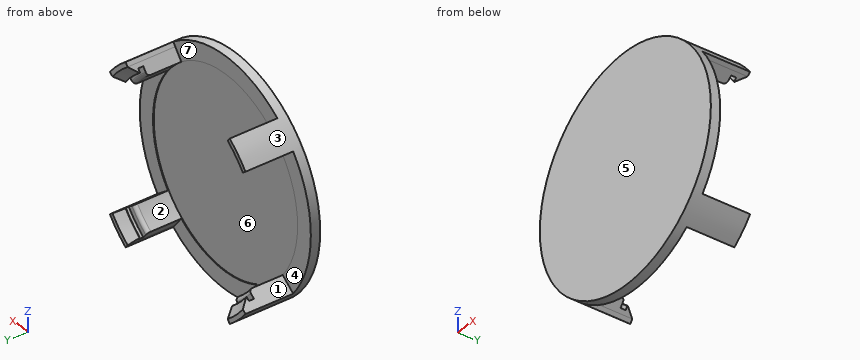
from build123d import *

# Parameters (mm, degrees)
CUT_EXTRUDE3_DEPTH = 17.4625
FILLET1_R          = 0.127
FILLET2_R          = 1.27


with BuildPart() as part:
    # Sketch1 → Revolve1 (revolve)
    with BuildSketch(Plane.XY):
        Polygon((0, 0), (-41.148, 0), (-41.148, 20.8915), (-39.5605, 20.8915), (-36.3855, 17.7165), (-37.973, 17.7165), (-37.973, 15.875), (-34.798, 15.875), (-34.798, 3.175), (0, 3.175), align=None)
    revolve(axis=Axis((0, 3.175, 0), (0, -1, 0)))

    # Sketch2 → Cut-Extrude3 (cut)
    with BuildSketch(Plane(origin=(0, 20.8915, 0), x_dir=(1, 0, 0), z_dir=(0, 1, 0))):
        with BuildLine():
            Line((-24.082906512, 31.385454819), (0, 0))
            Line((0, 0), (24.082906512, 31.385454819))
            ThreePointArc((24.082906512, 31.385454819), (0, 39.5605), (-24.082906512, 31.385454819))
        make_face()
        with BuildLine():
            Line((-25.049315281, 32.644903246), (-24.082906512, 31.385454819))
            ThreePointArc((-24.082906512, 31.385454819), (0, 39.5605), (24.082906512, 31.385454819))
            Line((24.082906512, 31.385454819), (25.049315281, 32.644903246))
            ThreePointArc((25.049315281, 32.644903246), (0, 41.148), (-25.049315281, 32.644903246))
        make_face()
        with BuildLine():
            Line((31.385454819, 24.082906512), (0, 0))
            Line((0, 0), (31.385454819, -24.082906512))
            ThreePointArc((31.385454819, -24.082906512), (37.461029388, -12.716305967), (39.5605, 0))
            ThreePointArc((39.5605, 0), (37.461029388, 12.716305967), (31.385454819, 24.082906512))
        make_face()
        with BuildLine():
            Line((32.644903246, 25.049315281), (31.385454819, 24.082906512))
            ThreePointArc((31.385454819, 24.082906512), (37.461029388, 12.716305967), (39.5605, 0))
            ThreePointArc((39.5605, 0), (37.461029388, -12.716305967), (31.385454819, -24.082906512))
            Line((31.385454819, -24.082906512), (32.644903246, -25.049315281))
            ThreePointArc((32.644903246, -25.049315281), (38.964280968, -13.226591118), (41.148, 0))
            ThreePointArc((41.148, 0), (38.964280968, 13.226591118), (32.644903246, 25.049315281))
        make_face()
        with BuildLine():
            Line((24.082906512, -31.385454819), (0, 0))
            Line((0, 0), (-24.082906512, -31.385454819))
            ThreePointArc((-24.082906512, -31.385454819), (0, -39.5605), (24.082906512, -31.385454819))
        make_face()
        with BuildLine():
            Line((25.049315281, -32.644903246), (24.082906512, -31.385454819))
            ThreePointArc((24.082906512, -31.385454819), (0, -39.5605), (-24.082906512, -31.385454819))
            Line((-24.082906512, -31.385454819), (-25.049315281, -32.644903246))
            ThreePointArc((-25.049315281, -32.644903246), (0, -41.148), (25.049315281, -32.644903246))
        make_face()
        with BuildLine():
            Line((0, 0), (-32.644903246, 25.049315281))
            ThreePointArc((-32.644903246, 25.049315281), (-41.148, 0), (-32.644903246, -25.049315281))
            Line((-32.644903246, -25.049315281), (0, 0))
        make_face()
    extrude(amount=-CUT_EXTRUDE3_DEPTH, mode=Mode.SUBTRACT)

    # Fillet1
    fillet1_edges = [part.edges().sort_by_distance(p)[0] for p in [
        (25.728433787, 17.7165, -25.728433787),
        (25.728433787, 17.7165, 25.728433787),
        (-25.728433787, 17.7165, 25.728433787),
        (-25.728433787, 17.7165, -25.728433787),
    ]]
    fillet(fillet1_edges, radius=FILLET1_R)

    # Fillet2
    fillet2_edges = [part.edges().sort_by_distance(p)[0] for p in [
        (24.605901772, 15.875, -24.605901772),
        (24.605901772, 15.875, 24.605901772),
        (-24.605901772, 15.875, 24.605901772),
        (-24.605901772, 15.875, -24.605901772),
    ]]
    fillet(fillet2_edges, radius=FILLET2_R)


solid = part.part
Could you check a few things on this model? Use its own coordinates, in mm. Face numbers are marked on the shaded views. A direction names the side the tool comes from. Coordinates: 2 decimals unless noted, no trailing zeros. Write each loop counter-clockwise with the first axis right and the second up, starting at its lowest first coordinate (ties: lowest second). Pieces come first, ordered by that corner, then holes. Notation, with made-up numbers: M -10.5,11 L 8.5,11 A25 ccw 8.5,34 Z; hole C 64,41.25 d9. An arc over 180 degrees is marked long. One line per question, with ' | ' between items.
1) I need wall thicknesses on probe 1 along Y at (x, z) = (4, -21.5) (3 decimals); probe 2 along Y at (x, z) = (-37, 3.5); probe 3 along Z at (x, y) = (32, 10.25). Which ranges of each line are inside material? Lowest first, please. Write a range as [from, to].
Checks:
probe 1: [0, 3.175] | probe 2: [0, 3.43] | probe 3: [-25.87, -24.55], [24.55, 25.87]
2) If we mould it in two halves opening along X, with no side actions, what happens to the marked faces 1, 2 and 3? For each: released by +X, released by -X, zero draft, split by the parting line, or undercut.
Checks:
face 1: released by -X | face 2: undercut | face 3: split by the parting line
3) Imagine slicing it at A-A, the plane y = 11.5. Write out the boundary of the cut face in (x, z).
Checks:
outline: M -32.64,-25.05 A41.15 ccw -25.05,-32.64 L -21.18,-27.61 A34.8 cw -27.61,-21.18 Z; M -32.64,25.05 L -27.61,21.18 A34.8 cw -21.18,27.61 L -25.05,32.64 A41.15 ccw Z; M 21.18,-27.61 L 25.05,-32.64 A41.15 ccw 32.64,-25.05 L 27.61,-21.18 A34.8 cw Z; M 21.18,27.61 A34.8 cw 27.61,21.18 L 32.64,25.05 A41.15 ccw 25.05,32.64 Z
4) For pin 1 Ø2.5 at (x, z) = (-27.5, 26) entering from +Y; pin 2 Ø15 at (x, z) = (32, -12) entering from +Y; pin 3 Ø5 at (x, y) = (-27, 15) entering from +Z, each with a flat end and sliding along its axis, tell me the tip position at first contact or that it passes through.
Checks:
pin 1: y = 20.43 | pin 2: y = 3.43 | pin 3: z = 32.64
5) Imagine slicing it at B-B, the plane x = 0. Write out the boundary of the cut face in (y, z) (3 decimals), and give its area (3 significant figures).
Checks:
outline: M 0,-41.148 L 3.429,-41.148 L 3.429,-34.798 L 3.175,-34.798 L 3.175,34.798 L 3.429,34.798 L 3.429,41.148 L 0,41.148 Z | area: 265 mm²
6) For the marked faces 4, 5, 6 and 7, which set-ups out of +Z, -Z, +X, -X, +Y, -Y let a thin tool reach every point of the face, with its end or its side?
Checks:
face 4: -X, +Y | face 5: +Z, -Z, +X, -X, -Y | face 6: +Y | face 7: +Z, +Y
7) Imagine slicing it at C-C, the plane z = 0. Write out the boundary of the cut face in (x, y) (3 decimals).
Checks:
outline: M -41.148,0 L 41.148,0 L 41.148,3.429 L 34.798,3.429 L 34.798,3.175 L -34.798,3.175 L -34.798,3.429 L -41.148,3.429 Z
